```python
from build123d import *

# Parameters (mm, degrees)
EXTRUDE_1_DEPTH = 1.25


with BuildPart() as part:
    # 草图2 → 凸台-拉伸1 (new body)
    with BuildSketch(Plane(origin=(0, 0, 0), x_dir=(1, 0, 0), z_dir=(0, 1, 0))):
        with BuildLine():
            Line((-15.5, 6.5), (15.5, 6.5))
            ThreePointArc((15.5, 6.5), (16.560660172, 6.060660172), (17, 5))
            Line((17, 5), (17, 0))
            Line((17, 0), (14, 0))
            ThreePointArc((14, 0), (13.707106781, 0.707106781), (13, 1))
            Line((13, 1), (11, 1))
            ThreePointArc((11, 1), (10.292893219, 0.707106781), (10, 0))
            Line((10, 0), (2.6, 0))
            ThreePointArc((2.6, 0), (0, 2.6), (-2.6, 0))
            Line((-2.6, 0), (-10, 0))
            ThreePointArc((-10, 0), (-10.292893219, 0.707106781), (-11, 1))
            Line((-11, 1), (-13, 1))
            ThreePointArc((-13, 1), (-13.707106781, 0.707106781), (-14, 0))
            Line((-14, 0), (-17, 0))
            Line((-17, 0), (-17, 5))
            ThreePointArc((-17, 5), (-16.560660172, 6.060660172), (-15.5, 6.5))
        make_face()
    extrude(amount=EXTRUDE_1_DEPTH)


solid = part.part
```
Geometry: final body of the model. Coordinates: model frame, mm. A direction names the side the tool comes from. Give positions to 0.01 mm unless a question says otherwise; leave off trailing zeros. Loops run counter-clockwise (first coordinate to the right, second up) from the corner with the lowest first, then second, coordinate; pieces in that order, holes last. Notation, with made-up numbers: (-31, 13.25) -> (17, 13.25) arc R22 ccw to (17, 30.25) -> close; hole circle Ø4 at (23, 45.5). An arc over 180 degrees is marked (long way). Use CSV: the item, a comma, the result in double quotes.
(1) Cut plane B-B (x = 0). Output: boundary loops of the cut face in (y, z), plus the area to 4 significant figures.
From the geometry:
outline,"(0, -6.5) -> (1.25, -6.5) -> (1.25, -2.6) -> (0, -2.6) -> close"
area,"4.875 mm^2"
(2) First-contact query: P1, Ø0.6, axis at x = -11.5, y = 0.5, coming from the +Z side. Flat tip, straight axial feed; report the tip coordinate or a pass-through.
From the geometry:
P1,"z = -1"
(3) Access query for faces 1 (the face through (-13.699, 0.616, -0.715)), 2 (the face through (0, 1.25, -3)). Directions: +Z, -Z, +X, -X, +Y, -Y. A direction counts if a zero-diameter tool reaches every point of the face in a straight line with its end or side. Return the directions, or none.
From the geometry:
face 1,"+Z, +Y, -Y"
face 2,"+Z, -Z, +X, -X, +Y"
(4) Ray query, line 1 along Z through (x, y) = (12, 0.35); line 2 along X through (y, z) = (0.7, -1.25); line 3 along X through (y, z) = (1.05, -1.5). Return the intervals inside material, ascending. Write a range as [from, to].
From the geometry:
line 1,"[-6.5, -1]"
line 2,"[-17, -2.28], [2.28, 17]"
line 3,"[-17, -2.12], [2.12, 17]"
(5) Cut plane A-A (y = 0.4). Output: boundary loops of the cut face in (x, z).
From the geometry:
outline,"(-17, -5) arc R1.5 ccw to (-15.5, -6.5) -> (15.5, -6.5) arc R1.5 ccw to (17, -5) -> (17, 0) -> (14, 0) arc R1 cw to (13, -1) -> (11, -1) arc R1 cw to (10, 0) -> (2.6, 0) arc R2.6 cw to (-2.6, 0) -> (-10, 0) arc R1 cw to (-11, -1) -> (-13, -1) arc R1 cw to (-14, 0) -> (-17, 0) -> close"
